from build123d import *

# Parameters (mm, degrees)
Y_KSEKLIK_EKSTR_ZYON1_DEPTH = 2
IZIM3_R                     = 1.5
KES_EKSTR_ZYON1_DEPTH       = 3
IZIM5_R                     = 1.5
KES_EKSTR_ZYON2_DEPTH       = 2


with BuildPart() as part:
    # Çizim1 → Yükseklik-Ekstrüzyon1 (new body)
    with BuildSketch(Plane.XY):
        with BuildLine():
            Line((-2.5, 50), (-2.5, 0))
            ThreePointArc((-2.5, 0), (0, -2.5), (2.5, 0))
            Line((2.5, 0), (2.5, 50))
            ThreePointArc((2.5, 50), (0, 52.5), (-2.5, 50))
        make_face()
    extrude(amount=-Y_KSEKLIK_EKSTR_ZYON1_DEPTH)

    # Çizim3 → Kes-Ekstrüzyon1 (cut, through all)
    with BuildSketch(Plane.XY):
        Circle(IZIM3_R)
    extrude(amount=-KES_EKSTR_ZYON1_DEPTH, mode=Mode.SUBTRACT)

    # Çizim5 → Kes-Ekstrüzyon2 (cut)
    with BuildSketch(Plane.XY):
        with Locations((0, 50)):
            Circle(IZIM5_R)
    extrude(amount=-KES_EKSTR_ZYON2_DEPTH, mode=Mode.SUBTRACT)


solid = part.part
Input: part model. Units: mm. Frame: model coordinates. Coordinates: 2 decimals unless noted, no trailing zeros. Order: outer loops, then holes, each group sorted by start corner. A loop starts at its lowest first (then second) coordinate and runs counter-clockwise, first axis right, second up. Notation, with made-up numbers: M -1.5,13.5 L 13.5,13.5 A29 cw 13.5,48.5 Z; hole C 79.25,43 d1. An arc over 180 degrees is marked long. Write item = value, one per line. Start each with the question number.
(1) Line query: line 1 along Y through (x, z) = (0, -0.9); line 2 along Y through (x, z) = (-0.55, -0.1); line 3 along Y through (x, z) = (1.6, -1.4). Output: solid intervals per line, ascending. Write a range as [from, to].
(2) Pull-direction query (Y, two-part tool) for faces 1 (the flat face through (0, 25, 0)), 2 (the cylindrical face through (-0.325, 48.536, -0.986)), 3 (the cylindrical face through (-0.1, -2.5, -1)); classes: released by +Y, released by -Y, zero draft, split by the parting line, or undercut.
(3) Section A-A on x = 0. Output: boundary loops of the cut face in (y, z), and give its area (3 significant figures).
(4) Section B-B on z = -1.1. Output: boundary loops of the cut face in (x, y).
(5) First-contact query: P1, Ø1, axis at x = 0.5, z = -1, coming from the -Y side. Flat tip, straight axial feed; report the tip coordinate or a pass-through.
Result set:
q1.line_1 = [-2.5, -1.5], [1.5, 48.5], [51.5, 52.5]
q1.line_2 = [-2.44, -1.4], [1.4, 48.6], [51.4, 52.44]
q1.line_3 = [-1.92, 51.92]
q2.face_1 = zero draft
q2.face_2 = undercut
q2.face_3 = released by -Y
q3.outline = M -2.5,-2 L -1.5,-2 L -1.5,0 L -2.5,0 Z; M 1.5,-2 L 48.5,-2 L 48.5,0 L 1.5,0 Z; M 51.5,-2 L 52.5,-2 L 52.5,0 L 51.5,0 Z
q3.area = 98.0 mm²
q4.outline = M -2.5,0 A2.5 ccw 2.5,0 L 2.5,50 A2.5 ccw -2.5,50 Z; hole C 0,0 d3; hole C 0,50 d3
q5.P1 = -2.5
